Job drawing, mm, ordinate dimensions from the low corner. One solid piece. Round coordinates to 2 decimals unless told otherwise and drop trailing zeros. Loops run counter-clockwise (first coordinate to the right, second up) from the corner with the lowest first, then second, coordinate; pieces in that order, holes last.
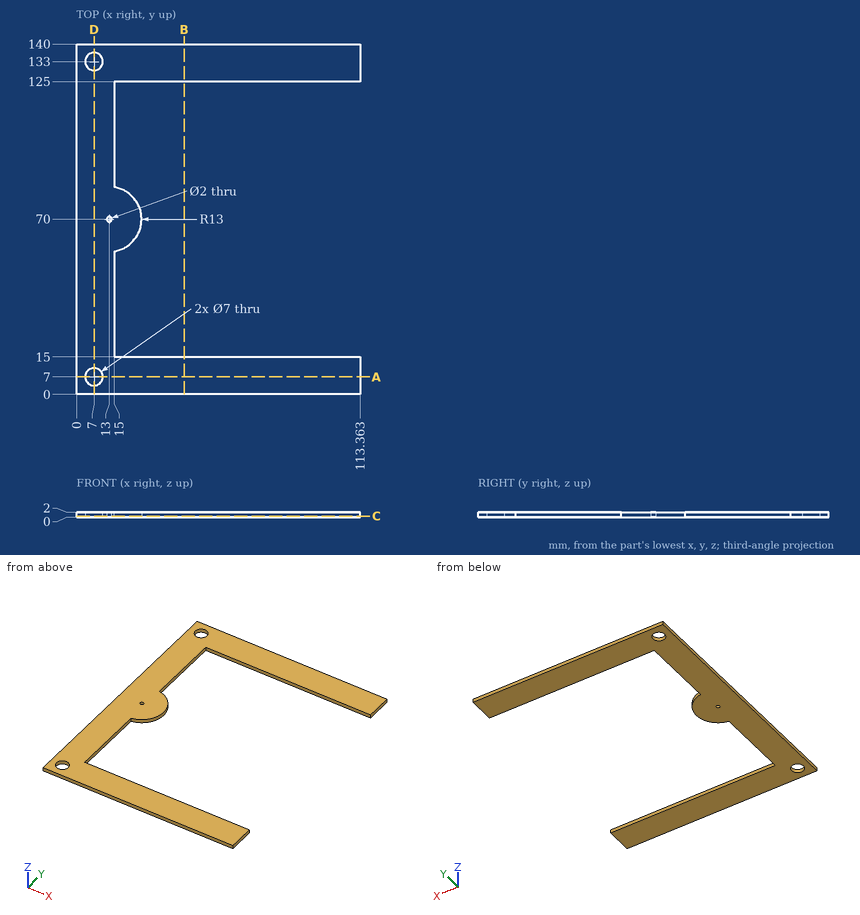
(1) Slice it at C-C on z = 0.5. List the corners of the cut face in (x, y) (1 decimal), plus the area to 3 significant figures.
Responses:
outline: (0, 0) - (113.4, 0) - (113.4, 15) - (15, 15) - (15, 57.2) arc R13 ccw to (15, 82.8) - (15, 125) - (113.4, 125) - (113.4, 140) - (0, 140) - close; hole circle Ø7 at (7, 7); hole circle Ø7 at (7, 133); hole circle Ø2 at (13, 70)
area: 5,180 mm2
(2) Slice it at A-A on y = 7. List the corners of the cut face in (x, z), plus the area to 3 significant figures.
Responses:
outline: (0, 0) - (3.5, 0) - (3.5, 2) - (0, 2) - close; (10.5, 0) - (113.36, 0) - (113.36, 2) - (10.5, 2) - close
area: 213 mm2
(3) Probe line 1 (Y direction, x = 7, z = 0.8); line 2 (Y direction, x = 92, z = 1.8); line 3 (X direction, y = 70, z = 0.75). List the from-to ranges inside material, lowest first.
Responses:
line 1: y = 0 to 3.5, 10.5 to 129.5, 136.5 to 140
line 2: y = 0 to 15, 125 to 140
line 3: x = 0 to 12, 14 to 26
(4) Slice it at D-D on x = 7. List the corners of the cut face in (y, z), plus the area to 3 significant figures.
Responses:
outline: (0, 0) - (3.5, 0) - (3.5, 2) - (0, 2) - close; (10.5, 0) - (129.5, 0) - (129.5, 2) - (10.5, 2) - close; (136.5, 0) - (140, 0) - (140, 2) - (136.5, 2) - close
area: 252 mm2
(5) Slice it at B-B on x = 43. List the corners of the cut face in (y, z).
Responses:
outline: (0, 0) - (15, 0) - (15, 2) - (0, 2) - close; (125, 0) - (140, 0) - (140, 2) - (125, 2) - close
